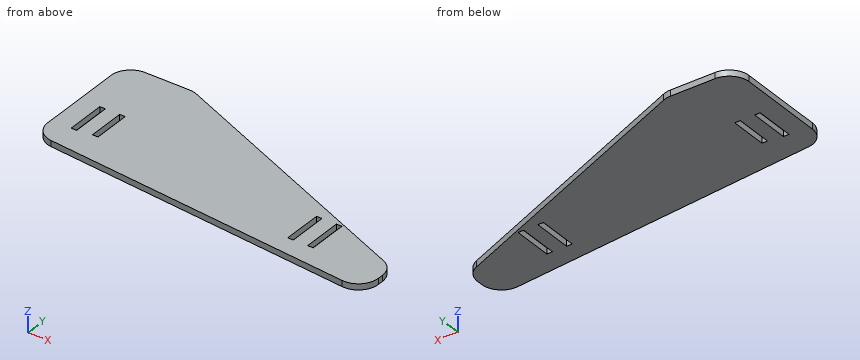
```python
from build123d import *

# Parameters (mm, degrees)
SKETCH2_W           = 2.8
SKETCH2_H           = 20
SKETCH2_H_2         = 20.000000002
SKETCH2_H_3         = 18.952705736
BOSS_EXTRUDE1_DEPTH = 3
FILLET1_R           = 10
SKETCH3_W           = 34.524922621
SKETCH3_H           = 4
CUT_EXTRUDE1_DEPTH  = 10
FILLET2_R           = 10


with BuildPart() as part:
    # Sketch2 → Boss-Extrude1 (new body)
    with BuildSketch(Plane.XY):
        Polygon((-20, 103.817072851), (5, 103.817072851), (157.9, 39.606577468), (157.9, 19.126615409), (-20, 36.779238836), align=None)
        with Locations((111.5, 43.194495368)):
            Rectangle(SKETCH2_W, SKETCH2_H, mode=Mode.SUBTRACT)
        with Locations((121.5, 43.194495368)):
            Rectangle(SKETCH2_W, SKETCH2_H, mode=Mode.SUBTRACT)
        with Locations((-8.5, 58.194495367)):
            Rectangle(SKETCH2_W, SKETCH2_H_2, mode=Mode.SUBTRACT)
        with Locations((1.5, 58.7181425)):
            Rectangle(SKETCH2_W, SKETCH2_H_3, mode=Mode.SUBTRACT)
    extrude(amount=BOSS_EXTRUDE1_DEPTH)

    # Fillet1
    fillet1_edges = [part.edges().sort_by_distance(p)[0] for p in [
        (157.9, 39.606577468, 1.5),
        (157.9, 19.126615409, 1.5),
        (-20, 36.779238836, 1.5),
    ]]
    fillet(fillet1_edges, radius=FILLET1_R)

    # Sketch3 → Cut-Extrude1 (cut)
    with BuildSketch(Plane(origin=(0, 0, 0), x_dir=(-1, 0, 0), z_dir=(0, 0, -1))):
        with Locations((2.737538689, 101.817072851)):
            Rectangle(SKETCH3_W, SKETCH3_H)
    extrude(amount=-CUT_EXTRUDE1_DEPTH, mode=Mode.SUBTRACT)

    # Fillet2
    fillet2_edges = [part.edges().sort_by_distance(p)[0] for p in [
        (14.524922621, 99.817072851, 1.5),
        (-20, 99.817072851, 1.5),
    ]]
    fillet(fillet2_edges, radius=FILLET2_R)


solid = part.part
```
Work out the finished part from the listing and answer in its coordinate system (mm). Give positions to 0.01 mm unless a question says otherwise; leave off trailing zeros. Loops run counter-clockwise (first coordinate to the right, second up) from the corner with the lowest first, then second, coordinate; pieces in that order, holes last. Notation, with made-up numbers: (26.5, 88) - (32.5, 88) arc R38 ccw to (32.5, 127) - close; hole circle Ø11 at (65, 66). An arc over 180 degrees is marked (long way). One line per question, with ' | ' between items.
(1) The part is cut by section B-B (y = 63.5). Write down the section's boundary in (x, z).
Recorded:
outline: (-20, 0) - (-9.9, 0) - (-9.9, 3) - (-20, 3) - close; (-7.1, 0) - (0.1, 0) - (0.1, 3) - (-7.1, 3) - close; (2.9, 0) - (101, 0) - (101, 3) - (2.9, 3) - close
(2) Straight lines are drawn through the part: probe 1 along X at (y, z) = (62.5, 1.6); probe 2 along X at (y, z) = (39, 0.95); probe 3 along Y at (x, z) = (112.5, 2.9). For each, find the intervals that lie inside material, in ascending order.
Recorded:
probe 1: x = -20 to -9.9, -7.1 to 0.1, 2.9 to 103.39 | probe 2: x = -17.3 to 110.1, 112.9 to 120.1, 122.9 to 155.87 | probe 3: y = 23.63 to 33.19, 53.19 to 58.67
(3) Each of these flat-tipped pins is pushed along its axis until it touches: pin 1 Ø0.9 at (y, z) = (38, 1.5) entering from +X; pin 2 Ø0.9 at (y, z) = (54.5, 1) entering from +X; pin 3 Ø0.8 at (x, z) = (2, 1.5) entering from -Y. Where does it stop, or does it pass through?
Recorded:
pin 1: stops at x = 156.78 | pin 2: stops at x = 123.51 | pin 3: stops at y = 34.56
(4) The part is cut by section A-A (z = 0.9). Write down the section's boundary in (x, y).
Recorded:
outline: (-20, 45.84) arc R10 ccw to (-10.99, 35.88) - (146.91, 20.22) arc R10 ccw to (157.9, 30.17) - (157.9, 32.96) arc R10 ccw to (151.77, 42.18) - (16.38, 99.04) arc R10 ccw to (12.51, 99.82) - (-10, 99.82) arc R10 ccw to (-20, 89.82) - close; hole (-9.9, 48.19) - (-7.1, 48.19) - (-7.1, 68.19) - (-9.9, 68.19) - close; hole (0.1, 49.24) - (2.9, 49.24) - (2.9, 68.19) - (0.1, 68.19) - close; hole (110.1, 33.19) - (112.9, 33.19) - (112.9, 53.19) - (110.1, 53.19) - close; hole (120.1, 33.19) - (122.9, 33.19) - (122.9, 53.19) - (120.1, 53.19) - close
(5) The part is cut by section C-C (x = 28). Write down the section's boundary in (y, z), then the cut area to 3 significant figures.
Recorded:
outline: (32.02, 0) - (94.16, 0) - (94.16, 3) - (32.02, 3) - close | area: 186 mm²
(6) The part is cut by section D-D (y = 82). Write down the section's boundary in (x, z), then the cut area to 3 significant figures.
Recorded:
outline: (-20, 0) - (56.95, 0) - (56.95, 3) - (-20, 3) - close | area: 231 mm²
